Geometry: final body of the model. Coordinates: model frame, mm. Face numbers are marked on the shaded views. A direction names the side the tool comes from. Round coordinates to 2 decimals unless told otherwise and drop trailing zeros. Loops run counter-clockwise (first coordinate to the right, second up) from the corner with the lowest first, then second, coordinate; pieces in that order, holes last. Notation, with made-up numbers: (89, -7) - (137, -7) arc R27 cw to (137, 31) - close; hole circle Ø6 at (75.5, 77.5). An arc over 180 degrees is marked (long way). Answer as a JSON object with one key per item and string values. Group by question number.
Item 1: Section A-A (z = 3.5). Return the cut outline in (x, y), plus the area to 3 significant figures.
Item 2: Draft query along X for the marked faces 1, 2 and 3. Return one class per face: released by +X, released by -X, zero draft, split by the parting line, or undercut.
Item 3: Line query: line 1 (Y direction, x = -0.35, z = 2.5); line 2 (Y direction, x = -0.25, z = 1); line 3 (Y direction, x = -0.8, z = 0.5). Output: solid intervals per line, ascending.
Item 4: Reachability of the marked faces 4 and 5 from +Z, -Z, +X, -X, +Y, -Y: full face, straight path, thin tool, end or side. Return the list, or none.
Item 5: First-contact query: pin 1 (1 mm diameter, centred on x = -0.5, z = 5, fed in from +Y); pin 2 (0.5 mm diameter, centred on y = 1, z = 0.5, fed in from -X); pin 3 (2 mm diameter, centred on y = -1, z = 6, fed in from +X). Flat tips, straight axial feed; report the tip coordinate or a pass-through.
Autodesk Inventor part; units mm, degrees
ref_plane "YZ Plane" through (0, 0, 0) normal (1, 0, 0) x (0, 1, 0)
ref_plane "XZ Plane" through (0, 0, 0) normal (0, 1, 0) x (-1, 0, 0)
ref_plane "XY Plane" through (0, 0, 0) normal (0, 0, 1) x (1, 0, 0)
sketch "スケッチ1" plane through (0, 0, 0) normal (1, 0, 0) x (0, 1, 0)
  line L0 (0, 7.7) -> (0, 0)
  line L1 (0, 0) -> (1.25, 0)
  line L2 (2.25, 1) -> (2.25, 1.7)
  line L3 (2.25, 1.7) -> (1.3, 1.7)
  line L4 (1.3, 1.7) -> (1.3, 7.7)
  line L5 (1.3, 7.7) -> (0, 7.7)
  line L6 (1.25, 0) -> (0, 1.7)
  arc A0 (1.25, 0) -> (2.25, 1) centre (1.25, 1) ccw
  line L7 (1.25, 0) -> (2.25, 0)
  line L8 (2.25, 0) -> (2.25, 1)
  dimension "d2" = 1.7
  dimension "d10" = 6
  dimension "d11" = 2.6
  dimension "d12" = 4.5
  dimension "d14" = 1
revolve "回転1" add sketch "スケッチ1" angle 360 about axis through (0, 0, 7.7) along (0, 0, -1) contours L5 L4 L3 L2 A0 L6 L0
thread "ねじ1"
sketch "スケッチ2" plane through (0, 0, 1.7) normal (0, 0, 1) x (1, 0, 0)
  line L0 (0.3339, -1.6357) -> (-0.3339, -1.6357)
  line L1 (-0.3339, -1.6357) -> (-0.3339, -0.7226)
  line L2 (-0.3339, 1.6357) -> (0.3339, 1.6357)
  line L3 (0.3339, 1.6357) -> (0.3339, 0.7226)
  line L4 (0.3339, -1.6357) -> (-0.3339, 1.6357) construction
  line L5 (-0.3339, -1.6357) -> (0.3339, 1.6357) construction
  line L6 (-1.5922, 0.2226) -> (-0.8339, 0.2226)
  line L7 (1.5922, 0.2226) -> (1.5922, -0.2226)
  line L8 (1.5922, -0.2226) -> (0.8339, -0.2226)
  line L9 (-1.5922, -0.2226) -> (-1.5922, 0.2226)
  line L10 (-1.5922, 0.2226) -> (1.5922, -0.2226) construction
  line L11 (1.5922, 0.2226) -> (-1.5922, -0.2226) construction
  circle A0 centre (0, 0) radius 2.25
  line L12 (0.3339, -0.7226) -> (0.3339, -1.6357)
  line L13 (0.8339, 0.2226) -> (1.5922, 0.2226)
  line L14 (-0.8339, -0.2226) -> (-1.5922, -0.2226)
  line L15 (-0.3339, 0.7226) -> (-0.3339, 1.6357)
  arc A1 (0.8339, -0.2226) -> (0.3339, -0.7226) centre (0.8339, -0.7226) ccw
  arc A2 (0.3339, 0.7226) -> (0.8339, 0.2226) centre (0.8339, 0.7226) ccw
  arc A3 (-0.8339, 0.2226) -> (-0.3339, 0.7226) centre (-0.8339, 0.7226) ccw
  arc A4 (-0.3339, -0.7226) -> (-0.8339, -0.2226) centre (-0.8339, -0.7226) ccw
  point P0 (0, 0)
  point P1 (-0.3339, -0.2226)
  point P2 (-0.3339, 0.2226)
  point P3 (0.3339, 0.2226)
  point P4 (0.3339, -0.2226)
  dimension "d18" = 0.5
extrude "押し出し2" add sketch "スケッチ2" against normal blind 1.7
revolve "回転2" cut sketch "スケッチ1" angle 360 about axis through (0, 0, 7.7) along (0, 0, -1) contours A0 L8 L7
properties part number "F-2606EB" material "チタン"
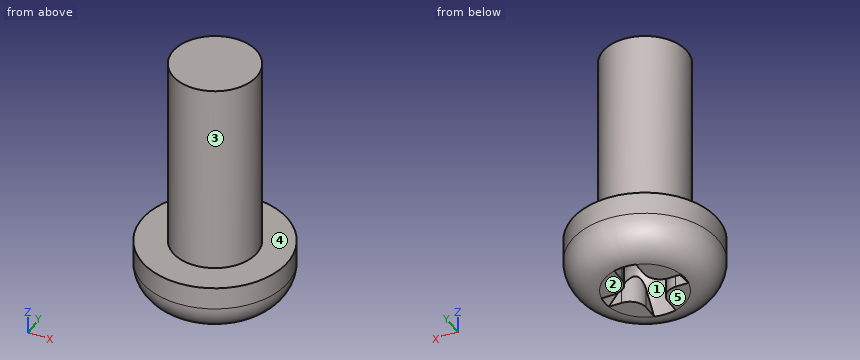
Values:
{
 "1": {"outline": "circle Ø2.6 at (0, 0)", "area": "5.31 mm^2"},
 "2": {"face 1": "undercut", "face 2": "zero draft", "face 3": "split by the parting line"},
 "3": {"line 1": "y = -1.25 to 1.25", "line 2": "y = -2.24 to -0.45, 0.45 to 2.24", "line 3": "y = -1.96 to -0.22, 0.22 to 1.96"},
 "4": {"face 4": "+Z", "face 5": "-Z, +X, -X, +Y, -Y"},
 "5": {"pin 1": "stops at y = 1.3", "pin 2": "stops at x = -2.04", "pin 3": "stops at x = 1.3"}
}
